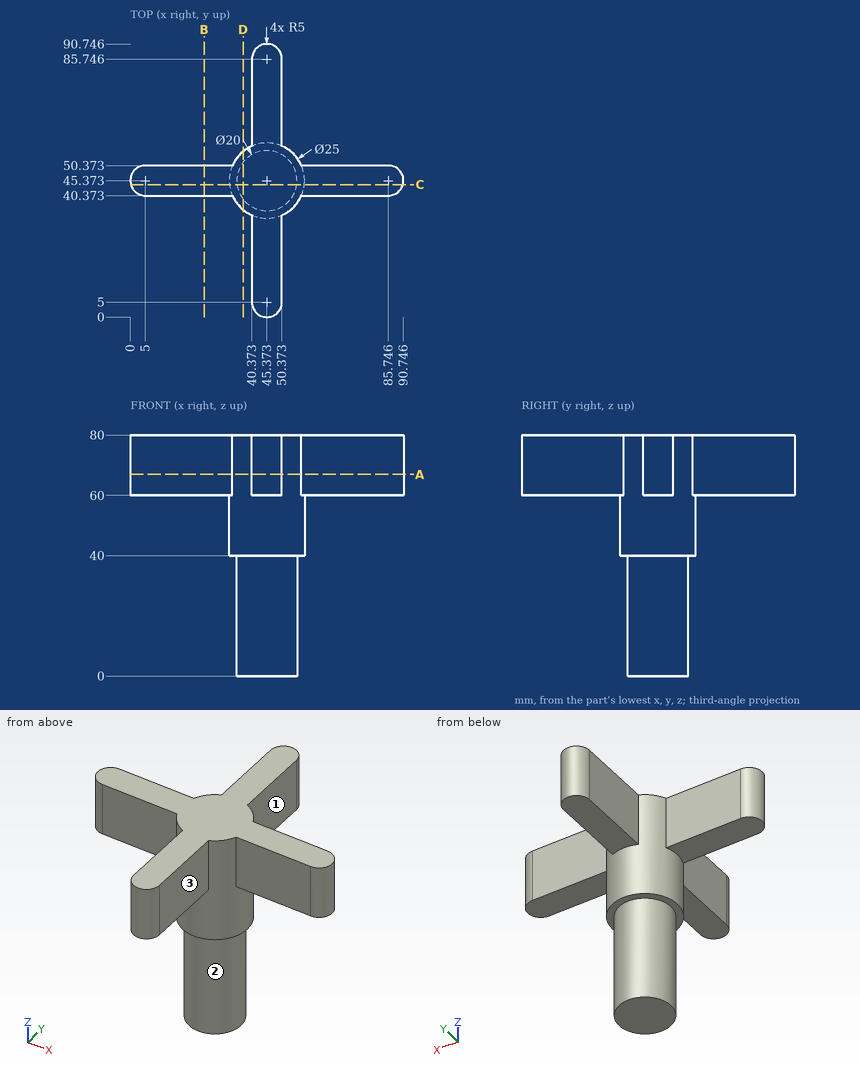
Verification items for this drawing (mm, ordinates from the low corner). A direction names the side the tool comes from. Coordinates: 2 decimals unless noted, no trailing zeros. Write each loop counter-clockwise with the first axis right and the second up, starting at its lowest first coordinate (ties: lowest second). Pieces come first, ordered by that corner, then holes. Notation, with made-up numbers: M 40,48 L 66,48 A12 cw 66,64 Z; hole C -38.75,61 d1. An arc over 180 degrees is marked long. One line per item, written item: value. Start each with the question number.
(1) Depth check by flat-ended pin: pin 1 (22 mm diameter, centred on x = 69, z = 68, fed in from -Y); pin 2 (5 mm diameter, centred on x = 44.5, y = 18.5, fed in from -Z); pin 3 (7.5 mm diameter, centred on x = 43, y = 50.5, fed in from -Z); pin 4 (10 mm diameter, centred on y = 21.5, z = 66.5, fed in from +X). Enter the tip coordinate at first touch or a pass-through.
(2) Scan lines: line 1 along Y through (x, z) = (33, 68); line 2 along Z through (x, y) = (44.5, 57). Record each from-to range of solid material in increasing order. Write a range as [from, to].
(3) Sectioned sample at B-B, the plane x = 24.5. Enter the section's corners in (y, z), and give its area (3 significant figures).
(4) Sectioned sample at A-A, the plane z = 67. Enter the section's corners in (x, y).
(5) Sectioned sample at D-D, the plane x = 37.5. Enter the section's corners in (y, z) (1 decimal).
(6) Tool access check on the marked faces 1, 2 and 3. Record the directions out of +Z, -Z, +X, -X, +Y, -Y that give a thin tool (end or side, any length) a straight path to the whole face; none if there is none.
(7) Sectioned sample at C-C, the plane y = 44. Enter the section's corners in (x, z).
Filled sheet:
1. pin 1: y = 40.37
1. pin 2: z = 60
1. pin 3: z = 0
1. pin 4: x = 50.37
2. line 1: [40.37, 50.37]
2. line 2: [40, 80]
3. outline: M 40.37,60 L 50.37,60 L 50.37,80 L 40.37,80 Z
3. area: 200 mm²
4. outline: M 5,40.37 L 33.92,40.37 A12.5 ccw 40.37,33.92 L 40.37,5 A5 ccw 50.37,5 L 50.37,33.92 A12.5 ccw 56.83,40.37 L 85.75,40.37 A5 ccw 85.75,50.37 L 56.83,50.37 A12.5 ccw 50.37,56.83 L 50.37,85.75 A5 ccw 40.37,85.75 L 40.37,56.83 A12.5 ccw 33.92,50.37 L 5,50.37 A5 ccw Z
5. outline: M 35.7,40 L 39.2,40 L 39.2,0 L 51.5,0 L 51.5,40 L 55.1,40 L 55.1,80 L 35.7,80 Z
6. face 1: +Z, -Z, +X, +Y
6. face 2: -Z
6. face 3: +Z, -Z, +X, -Y
7. outline: M 0.19,60 L 32.95,60 L 32.95,40 L 35.47,40 L 35.47,0 L 55.28,0 L 55.28,40 L 57.8,40 L 57.8,60 L 90.55,60 L 90.55,80 L 0.19,80 Z
